Work out the finished part from the listing and answer in its coordinate system (mm). A direction names the side the tool comes from. Round coordinates to 2 decimals unless told otherwise and drop trailing zeros. Loops run counter-clockwise (first coordinate to the right, second up) from the corner with the lowest first, then second, coordinate; pieces in that order, holes last.
```python
from build123d import *

# Parameters (mm, degrees)
SKETCH1_W           = 5
SKETCH1_H           = 30
BOSS_EXTRUDE1_DEPTH = 38.1
SKETCH2_W           = 2
SKETCH2_H           = 25.4
CUT_EXTRUDE1_DEPTH  = 151
BOSS_EXTRUDE3_DEPTH = 150
CUT_EXTRUDE2_START  = -145
SKETCH4_W           = 32.727499149
SKETCH4_H           = 37.13145561
CUT_EXTRUDE2_DEPTH  = 145


with BuildPart() as part:
    # Sketch1 → Boss-Extrude1 (new body)
    with BuildSketch(Plane(origin=(0, 0, 0), x_dir=(1, 0, 0), z_dir=(0, 1, 0))):
        with Locations((-72.5, -15)):
            Rectangle(SKETCH1_W, SKETCH1_H)
        with BuildLine():
            ThreePointArc((75, 0), (0, 75), (-75, 0))
            Line((-75, 0), (-70, 0))
            ThreePointArc((-70, 0), (0, 70), (70, 0))
            Line((70, 0), (75, 0))
        make_face()
        with Locations((72.5, -15)):
            Rectangle(SKETCH1_W, SKETCH1_H)
    extrude(amount=BOSS_EXTRUDE1_DEPTH)

    # Sketch2 → Cut-Extrude1 (cut, through all)
    with BuildSketch(Plane(origin=(75, 0, 0), x_dir=(0, 0, -1), z_dir=(1, 0, 0))):
        with Locations((-24, 19.05)):
            Rectangle(SKETCH2_W, SKETCH2_H)
    extrude(amount=-CUT_EXTRUDE1_DEPTH, mode=Mode.SUBTRACT)

    # Sketch3 → Boss-Extrude3 (add)
    with BuildSketch(Plane(origin=(75, 0, 0), x_dir=(0, 0, -1), z_dir=(1, 0, 0))):
        Polygon((0, -30), (-30, 0), (-30, -4), (-4, -30), align=None)
        with BuildLine():
            Line((-26.464466094, 0), (-30, 0))
            Line((-30, 0), (0, -30))
            Line((0, -30), (0, -26.464466094))
            Line((0, -26.464466094), (-3.213911245, -23.250554849))
            ThreePointArc((-3.213911245, -23.250554849), (-6.581507291, -23.250554849), (-6.581507291, -19.882958803))
            Line((-6.581507291, -19.882958803), (-20.891580775, -5.572885319))
            ThreePointArc((-20.891580775, -5.572885319), (-24.25917682, -5.572885319), (-24.25917682, -2.205289274))
            Line((-24.25917682, -2.205289274), (-26.464466094, 0))
        make_face()
        with BuildLine():
            Line((-22.928932188, 0), (-26.464466094, 0))
            Line((-26.464466094, 0), (-24.25917682, -2.205289274))
            ThreePointArc((-24.25917682, -2.205289274), (-21.664113874, -1.68909916), (-20.194128798, -3.889087297))
            ThreePointArc((-20.194128798, -3.889087297), (-20.375390661, -4.80035222), (-20.891580775, -5.572885319))
            Line((-20.891580775, -5.572885319), (-6.581507291, -19.882958803))
            ThreePointArc((-6.581507291, -19.882958803), (-3.986444345, -19.366768689), (-2.516459268, -21.566756826))
            ThreePointArc((-2.516459268, -21.566756826), (-2.697721131, -22.47802175), (-3.213911245, -23.250554849))
            Line((-3.213911245, -23.250554849), (0, -26.464466094))
            Line((0, -26.464466094), (0, -22.928932188))
            Line((0, -22.928932188), (-22.928932188, 0))
        make_face()
        Polygon((0, 0), (-22.928932188, 0), (0, -22.928932188), align=None)
    extrude(amount=-BOSS_EXTRUDE3_DEPTH)

    # Sketch4 → Cut-Extrude2 (cut)
    with BuildSketch(Plane(origin=(75, 0, 0), x_dir=(0, 0, -1), z_dir=(1, 0, 0)).offset(CUT_EXTRUDE2_START)):
        with Locations((-16.363749575, -18.565727805)):
            Rectangle(SKETCH4_W, SKETCH4_H)
    extrude(amount=CUT_EXTRUDE2_DEPTH, mode=Mode.SUBTRACT)


solid = part.part
```
1. Given pin 1 (1 mm diameter, centred on y = -12, z = 12, fed in from +X); pin 2 (12 mm diameter, centred on y = 29, z = -25, fed in from -X); pin 3 (1.6 mm diameter, centred on x = 73.5, z = 24.5, fed in from -Y), each flat-ended and moving along its own axis, determine where each tip first touches the part or whether it passes through.
Answer key:
pin 1: stops at x = -70
pin 2: stops at x = -72.55
pin 3: stops at y = 0
2. Find section D-D (z = -64). Write down the section's boundary in (x, y), then the cut area to 3 significant figures.
Answer key:
outline: (-39.1, 0) - (-28.35, 0) - (-28.35, 38.1) - (-39.1, 38.1) - close; (28.35, 0) - (39.1, 0) - (39.1, 38.1) - (28.35, 38.1) - close
area: 819 mm2
3. Determine the mould class of faces 4 (the face through (16, 0, -69)), 5 (the face through (73, 19, 23)), 6 (the face through (1.65, 18.78, -74.98)) for opening direction Z: +Z half, -Z half, draft (parallel to the pull), parting line (faces both ways), or undercut.
Answer key:
face 4: draft
face 5: undercut
face 6: -Z half
4. Consider probe 1 along X at (y, z) = (33, 4.5); probe 2 along X at (y, z) = (15, -39.5); probe 3 along Y at (x, z) = (51.5, -48). Determine where each line is inside the solid, lowest interval first.
Answer key:
probe 1: x = -75 to -70, 70 to 75
probe 2: x = -63.76 to -57.79, 57.79 to 63.76
probe 3: y = 0 to 38.1
5. Which of the six approach directions +Z, -Z, +X, -X, +Y, -Y give full straight-line access (tool end or side, diameter ignored) to faces 1 (the face through (-72, -15, 0)), 2 (the face through (-70, 11, 15)), 3 (the face through (-72, 19, 25))?
Answer key:
face 1: -Z, +X, -X, -Y
face 2: +Z, +Y, -Y
face 3: +X, -X
6. Find section B-B (z = -23). Write down the section's boundary in (x, y), then the cut area to 3 significant figures.
Answer key:
outline: (-71.39, 0) - (-66.11, 0) - (-66.11, 38.1) - (-71.39, 38.1) - close; (66.11, 0) - (71.39, 0) - (71.39, 38.1) - (66.11, 38.1) - close
area: 402 mm2
7. Find section C-C (x = 0). Write down the section's boundary in (y, z).
Answer key:
outline: (0, -75) - (38.1, -75) - (38.1, -70) - (0, -70) - close
8. Find section A-A (y = 9). Write down the section's boundary in (x, z), then the cut area to 3 significant figures.
Answer key:
outline: (-75, 0) arc R75 ccw to (75, 0) - (75, 23) - (70, 23) - (70, 0) arc R70 cw to (-70, 0) - (-70, 23) - (-75, 23) - close; (-75, 25) - (-70, 25) - (-70, 30) - (-75, 30) - close; (70, 25) - (75, 25) - (75, 30) - (70, 30) - close
area: 1,420 mm2
